```python
from build123d import *

# Parameters (mm, degrees)
F0_W     = 62.45
F0_H     = 62.4586
F1_DEPTH = 4
F2_R     = 2.9
F4_DEPTH = 10
F3_R     = 2.9
F5_DEPTH = 10
F6_W     = 62.45
F6_H     = 41.379086
F6_R     = 2.9
F7_DEPTH = 2.5


with BuildPart() as f1:
    # F0 (on Top) → F1 (new body)
    with BuildSketch(Plane.XY):
        with Locations((31.225, 31.2293)):
            Rectangle(F0_W, F0_H)
    extrude(amount=-F1_DEPTH)

    # F2 (on face) → F4 (join)
    with BuildSketch(Plane.XY):
        with Locations((6.025, 6.025)):
            Circle(F2_R)
        with Locations((56.425, 6.025)):
            Circle(F2_R)
    extrude(amount=F4_DEPTH)

    # F3 (on face) → F5 (join)
    with BuildSketch(Plane.XY):
        with Locations((56.425, 56.425)):
            Circle(F3_R)
        with Locations((6.025, 56.425)):
            Circle(F3_R)
    extrude(amount=F5_DEPTH)

    # F6 (on face) → F7 (join)
    with BuildSketch(Plane.XY):
        with Locations((31.225, 41.769057)):
            Rectangle(F6_W, F6_H)
        with Locations((6.025, 56.425)):
            Circle(F6_R, mode=Mode.SUBTRACT)
        with Locations((56.425, 56.425)):
            Circle(F6_R, mode=Mode.SUBTRACT)
    extrude(amount=F7_DEPTH)


solid = f1.part
```
Read the model definition and answer for the solid it produces. Units are mm, in the model's axes. A direction names the side the tool comes from. Coordinates: 2 decimals unless noted, no trailing zeros. Write each loop counter-clockwise with the first axis right and the second up, starting at its lowest first coordinate (ties: lowest second). Pieces come first, ordered by that corner, then holes. Notation, with made-up numbers: (-37.75, -3.75) -> (13.25, -3.75) arc R31 cw to (13.25, 35.25) -> close; hole circle Ø5 at (57.25, 36). An arc over 180 degrees is marked (long way). Write item = value, one per line.
(1) Section B-B on x = 11 is taken. Write down the section's boundary in (y, z).
From the geometry:
outline = (0, -4) -> (62.46, -4) -> (62.46, 2.5) -> (21.08, 2.5) -> (21.08, 0) -> (0, 0) -> close
(2) Which of the six approach directions +Z, -Z, +X, -X, +Y, -Y give full straight-line access (tool end or side, diameter ignored) to faces 1 (the face through (56, 6, 10)), 2 (the face through (57.984, 58.87, 6.198))?
From the geometry:
face_1 = +Z, +X, -X, +Y, -Y
face_2 = +Z
(3) Straight lines are drawn through the part: L1, parallel to Z at x = 3, y = 40; L2, parallel to X at y = 55, z = 5; L3, parallel to Z at x = 21, y = 7.5. For each, find the intervals that lie inside material, in ascending order. Write a range as from..to.
From the geometry:
L1 = -4..2.5
L2 = 3.5..8.55, 53.9..58.95
L3 = -4..0
(4) Given pin 1 Ø4 at (y, z) = (10, 5) entering from +X; pin 2 Ø0.8 at (x, z) = (32, 0.5) entering from -Y; pin 3 Ø17 at (x, y) = (41.5, 11) entering from +Z, each flat-ended and moving along its own axis, determine where each tip first touches the part or whether it passes through.
From the geometry:
pin_1 = 58.55
pin_2 = 21.08
pin_3 = 0
(5) Section C-C on y = 12 is taken. Write down the section's boundary in (x, z), plus the area to 3 significant figures.
From the geometry:
outline = (0, -4) -> (62.45, -4) -> (62.45, 0) -> (0, 0) -> close
area = 250 mm2
(6) Section A-A on z = 0.75 is taken. Write down the section's boundary in (x, y) (3 decimals), plus the area to 3 significant figures.
From the geometry:
outline = (0, 21.08) -> (62.45, 21.08) -> (62.45, 62.459) -> (0, 62.459) -> close; circle Ø5.8 at (6.025, 6.025); circle Ø5.8 at (56.425, 6.025)
area = 2,640 mm2
(7) For a pull along Y with two mould halves and no side action, classify faces 3 (the face through (31, 62.459, -1)), 4 (the face through (56, 56, 10)), 5 (the face through (59.19, 6.9, 4.93)) as +Y half, -Y half, draft (parallel to the pull), parting line (faces both ways), or undercut.
From the geometry:
face_3 = +Y half
face_4 = draft
face_5 = undercut
(8) Section D-D on x = 55 is taken. Write down the section's boundary in (y, z), plus the area to 3 significant figures.
From the geometry:
outline = (0, -4) -> (62.46, -4) -> (62.46, 2.5) -> (58.95, 2.5) -> (58.95, 10) -> (53.9, 10) -> (53.9, 2.5) -> (21.08, 2.5) -> (21.08, 0) -> (8.55, 0) -> (8.55, 10) -> (3.5, 10) -> (3.5, 0) -> (0, 0) -> close
area = 442 mm2
